Here's how the part is built. I have some questions about the finished solid (model axes, mm). Face numbers are marked on the shaded views. A direction names the side the tool comes from. Give positions to 0.01 mm unless a question says otherwise; leave off trailing zeros. Loops run counter-clockwise (first coordinate to the right, second up) from the corner with the lowest first, then second, coordinate; pieces in that order, holes last.
Q1. Suppose I cut it at C-C (y = 255). List the corners of the cut face in (x, z) for me.
Q2. I'm going to push flat-ended pins straight in: P1, Ø1, axis at x = -180.5, y = 371, coming from the -Z side; P2, Ø2, axis at x = 139.5, z = 0.5, coming from the -Y side; P3, Ø3, axis at x = 90.5, z = -14, coming from the +Y side. Where does each tip first touch, or does it pass through?
Q3. For the marked faces 1 and 2, which set-ups out of +Z, -Z, +X, -X, +Y, -Y let a thin tool reach every point of the face, with its end or its side?
Q4. Suppose I cut it at B-B (x = -28.5). List the corners of the cut face in (y, z) for me.
Q5. Suppose I cut it at A-A (z = 12). List the corners of the cut face in (x, y) for me, and give its area (3 significant figures).
Q6. I need wall thicknesses on probe 1 along Z at (x, y) = (127.5, -3.5); probe 2 along X at (y, z) = (140.5, 9.5); probe 3 along X at (y, z) = (292, 1.5). Which ranges of each line are inside material? Lowest first, please.
```python
from build123d import *

# Parameters (mm, degrees)
F1_DEPTH = 19.05
F3_DEPTH = 19.05


with BuildPart() as f1:
    # F0 (on Top) → F1 (new body)
    with BuildSketch(Plane.XY):
        Polygon((281.657545, 545.334344), (-334.292455, 545.334344), (-334.292455, 342.134344), (173.707545, -184.915656), (281.657545, -184.915656), align=None)
    extrude(amount=F1_DEPTH)

    # F2 (on face) → F3 (join)
    with BuildSketch(Plane(origin=(0, 0, 0), x_dir=(1, 0, 0), z_dir=(0, 0, -1))):
        Polygon((-334.292455, -342.134344), (-334.292455, -369.5849), (200.165912, 184.915656), (173.707545, 184.915656), align=None)
    extrude(amount=F3_DEPTH)


solid = f1.part
```
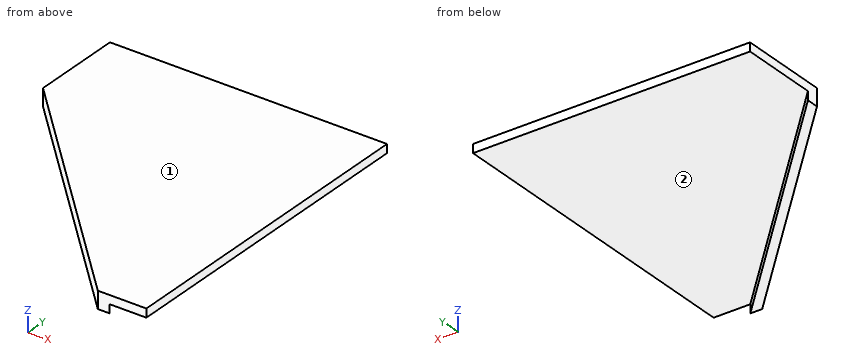
Solutions:
1. outline: (-250.31, -19.05) - (-223.85, -19.05) - (-223.85, 0) - (281.66, 0) - (281.66, 19.05) - (-250.31, 19.05) - close
2. P1: stops at z = 0
2. P2: stops at y = -150.46
2. P3: stops at y = -69.58
3. face 1: +Z, +X, -X, +Y, -Y
3. face 2: -Z, +X, +Y
4. outline: (24.87, -19.05) - (52.33, -19.05) - (52.33, 0) - (545.33, 0) - (545.33, 19.05) - (24.87, 19.05) - close
5. outline: (-334.29, 342.13) - (173.71, -184.92) - (281.66, -184.92) - (281.66, 545.33) - (-334.29, 545.33) - close
5. area: 316,000 mm2
6. probe 1: z = 0 to 19.05
6. probe 2: x = -139.95 to 281.66
6. probe 3: x = -285.97 to 281.66
